Answer from the drawing. Dimensions are ordinates in mm from the lowest x, y and z of the part. Give positions to 0.01 mm unless a question says otherwise; leave off trailing zeros. Loops run counter-clockwise (first coordinate to the right, second up) from the corner with the lowest first, then second, coordinate; pieces in that order, holes last.
(1) Straight lines are drawn through the part: probe 1 along Y at (x, z) = (35, 1.15) (1 decimal); probe 2 along Y at (x, z) = (9.5, 0.75) (1 decimal); probe 3 along X at (y, z) = (19.5, 1.5). For each, find the intervals that lie inside material, in ascending order.
(2) Find section B-B, the plane x = 39. Write down the section's boundary in (y, z) (1 decimal).
(3) Find section C-C, the plane y = 7. Write down the section's boundary in (x, z) (1 decimal).
(4) Find section A-A, the plane z = 0.8. State how many separate pieces and enclosed holes the cut face has, then the cut area to 3 significant figures.
(5) This flat-tipped pin is pushed along its axis until it touches: P1, Ø1.5, axis at x = 9.971, y = 8.828, coming from the -Z side. Where does it stop, or does it pass through?
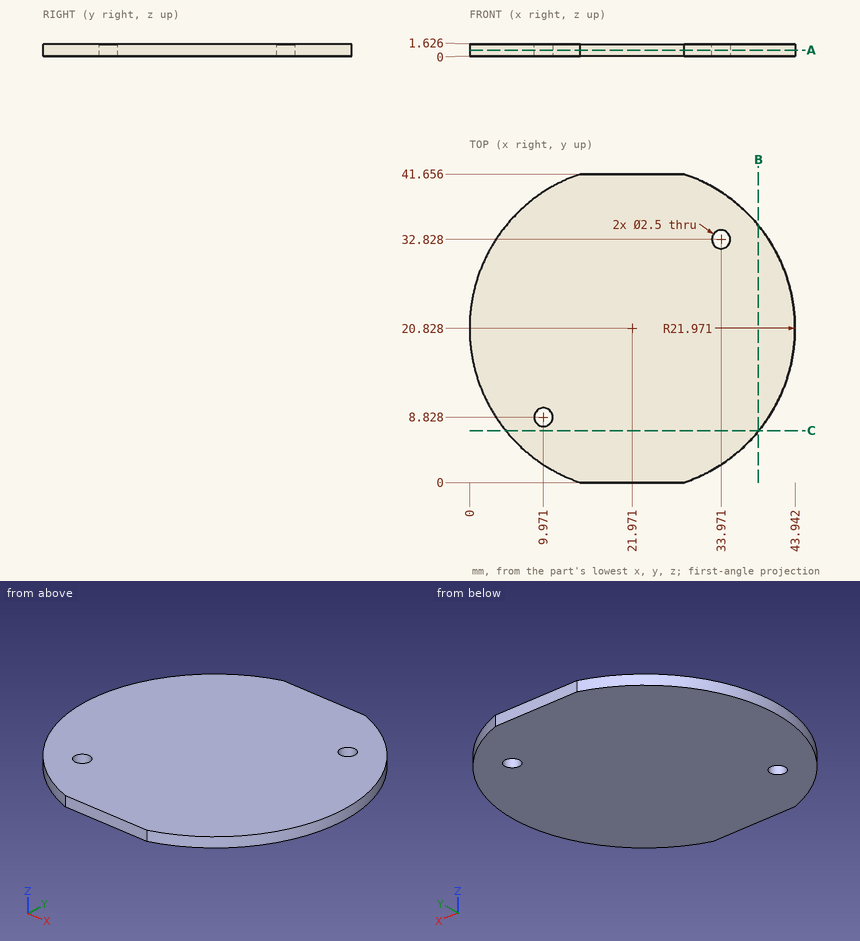
Entries:
1. probe 1: y = 3.1 to 32.1, 33.5 to 38.5
1. probe 2: y = 2.7 to 7.7, 10 to 38.9
1. probe 3: x = 0.04 to 43.9
2. outline: (6.9, 0) - (34.7, 0) - (34.7, 1.6) - (6.9, 1.6) - close
3. outline: (4.9, 0) - (39, 0) - (39, 1.6) - (4.9, 1.6) - close
4. separate pieces: 1
4. enclosed holes: 2
4. area: 1,490 mm2
5. P1: passes through
